Autodesk Inventor part; units mm, degrees
ref_plane "MSC_PT1" through (5.7, 0, 0) normal (1, 0, 0) x (0, 1, 0)
ref_plane "MSC_PT2" through (0, 0, 0) normal (-1, 0, 0) x (0, -1, 0)
ref_plane "MSC_PF1" through (0, 0, 0) normal (1, 0, 0) x (0, 1, 0)
sketch "Sketch1" plane through (0, 0, 0) normal (1, 0, 0) x (0, 1, 0)
  line L0 (5, 2.8868) -> (5, -2.8868)
  line L1 (5, -2.8868) -> (0, -5.7735)
  line L2 (0, -5.7735) -> (-5, -2.8868)
  line L3 (-5, -2.8868) -> (-5, 2.8868)
  line L4 (-5, 2.8868) -> (0, 5.7735)
  line L5 (0, 5.7735) -> (5, 2.8868)
  circle A0 centre (0, 0) radius 5 construction
  dimension "d0" = 10
extrude "Extrusion1" add sketch "Sketch1" along normal blind 5.7
sketch "Sketch2" plane through (5.7, 0, 0) normal (1, 0, 0) x (0, 1, 0)
  line L0 (-5, 2.8868) -> (0, 5.7735)
  line L1 (0, -5.7735) -> (-5, -2.8868)
  line L2 (-5, 2.8868) -> (5, -2.8868) construction
  line L3 (-5, -2.8868) -> (5, 2.8868) construction
  point P0 (0, 0)
hole "Hole1" at (5.7, 0, 0) direction (-1, 0, 0) diameter 4.917 end through all
chamfer "Chamfer1" distance 0.5 angle 45 2 edges at (5.7, 0, 2.4585) (0, 0, 2.4585)
sketch "Sketch3" plane through (0, 0, 0) normal (0, 1, 0) x (-1, 0, 0)
  line L0 (-7.0172, 0) -> (2.1698, 0)
  line L1 (-5.7048, 0) -> (0.8574, 0)
  line L2 (-5.7, 0) -> (-5.7, -5.7735)
  line L3 (-5.7, -5.7735) -> (0, -5.7735)
  line L4 (0, -5.7735) -> (0, 0)
  line L5 (-5.7, -2.8868) -> (-5.7, -5.7735)
  line L6 (0, -2.8868) -> (0, -5.7735)
  line L7 (0, -5.7735) -> (-5.7, -5.7735)
  line L8 (-5.7, -5) -> (-5.2534, -5.7735)
  line L9 (-5.7, -5.7735) -> (-5.7, -5)
  line L10 (-5.7, -5.7735) -> (-5.2534, -5.7735)
  line L11 (0, -5) -> (-0.4466, -5.7735)
  line L12 (-0.4466, -5.7735) -> (0, -5.7735)
  line L13 (0, -5.7735) -> (0, -5)
  dimension "d32" = 5
  dimension "d33" = 30
revolve "Revolution1" cut sketch "Sketch3" angle 360 about axis through (0, 0, 0) along (-1, 0, 0) contours L8 L3 L2 | L4 L3 L11
ref_plane "MSC_PT1" through (5.7, 0, 0) normal (1, 0, 0) x (0, 1, 0)
ref_plane "MSC_PT2" through (0, 0, 0) normal (-1, 0, 0) x (0, -1, 0)
ref_plane "MSC_PF1" through (0, 0, 0) normal (1, 0, 0) x (0, 1, 0)
equation "\"d0\" = Smax"
equation "\"d1\" = Mmax"
equation "\"d10\" = 0.5 * PTC"
equation "\"d32\" = 0.5 * Smax"
equation "\"NND\" = 6"
equation "\"Smax\" = 10"
equation "\"Mmax\" = 5.7"
equation "\"PTC\" = 1"
equation "\"THREADDIA\" = NND"
equation "\"TEMPLATE\" = 1.2345"
properties part number "ANSI B18.2.4.2M - M6x1" material "Steel, Mild"
Design review of the part built by this model. Coordinates are the model's own, in mm. Coordinates: 2 decimals unless noted, no trailing zeros. Write each loop counter-clockwise with the first axis right and the second up, starting at its lowest first coordinate (ties: lowest second). Pieces come first, ordered by that corner, then holes. Notation, with made-up numbers: M -39.5,21.5 L -25.5,21.5 A18 cw -25.5,46.5 Z; hole C 62,36 d10. An arc over 180 degrees is marked long. Answer as a JSON object with one key per item and string values.
Item 1: Add section A-A, the plane x = 1.9. Give the boundary of the cut face in (y, z).
Outcome:
{"outline": "M -5,-2.89 L 0,-5.77 L 5,-2.89 L 5,2.89 L 0,5.77 L -5,2.89 Z; hole C 0,0 d4.92"}
Item 2: Draft analysis for pull direction Z (two halves, no side actions). For faces 1 (the flat face through (3, -5, 0)), 2 (the cylindrical face through (2.817, -0.738, -2.345)), 3 (the conical face through (0.11, 4.5, 2.58)), state which applies: pulls with the +Z half, pulls with the -Z half, needs draft (parallel to the pull), parting line crosses it, or undercut.
Outcome:
{"face 1": "needs draft", "face 2": "undercut", "face 3": "pulls with the +Z half"}
Item 3: Wall thickness on probe 1 along Y at (x, z) = (4.25, 0); probe 2 along Z at (x, y) = (0.65, 1.5); probe 3 along Y at (x, z) = (3.55, -0.5): over which ranges is each line inside the solid? List them lowest first.
Outcome:
{"probe 1": "-5 to -2.46, 2.46 to 5", "probe 2": "-4.91 to -1.95, 1.95 to 4.91", "probe 3": "-5 to -2.41, 2.41 to 5"}
Item 4: Insertion check: pin 1 Ø1.5 at (x, y) = (4.5, -1) entering from -Z. The pin has a flat end and moves straight along its axis. Give the tip position at first contact, or say it passes through.
Outcome:
{"pin 1": "z = -5.63"}
